For this review, take the finished solid that the model builds, in its own axes (mm). Face numbers are marked on the shaded views. A direction names the side the tool comes from. Give positions to 0.01 mm unless a question says otherwise; leave off trailing zeros. Order: outer loops, then holes, each group sorted by start corner. A loop starts at its lowest first (then second) coordinate and runs counter-clockwise, first axis right, second up. Notation, with made-up numbers: (-0.75, -1) - (14.25, -1) arc R8 cw to (14.25, 11) - close; hole circle Ø7 at (-2, 9). An arc over 180 degrees is marked (long way). Use a Markdown table: item, result. Add a question column.
1) We need section D-D on y = 2.5. Write out the cut boundary in (x, z).
2) We need section A-A on y = -52. Write out the cut boundary in (x, z).
3) Mouldability with a two-part tool opening along Y and no side actions: class the marked faces 1, 2 and 3 as released by +Y, released by -Y, zero draft, split by the parting line, or undercut.
4) Machinability: for the marked faces 4, 5 and 6, which of the approach directions +Z, -Z, +X, -X, +Y, -Y give a long, thin tool a straight path to every point of the face, cutting with its end or side? Answer none if there is none.
5) We need section C-C on z = 10.5. Write out the cut boundary in (x, y).
6) Wall thickness on L1, parallel to Y at x = 96.5, z = 22.5; L2, parallel to Y at x = 90.5, z = 23.5; L3, parallel to X at y = 152.5, z = 9.5: over which ranges is each line inside the solid? List them lowest first.
7) Clearance check with flat-ended pins moving along their axes: P1, Ø10, axis at y = 51, z = 108.5, coming from the +X side; P2, Ø1, axis at y = 103.5, z = 56, coming from the -X side; P3, Ø3, axis at x = 101.5, z = 52.5, coming from the -Y side; P4, Ø1.5, axis at x = 154.5, y = 118.5, coming from the +Z side. State where each tip first meets the part, or that it passes through.
8) We need section B-B on x = 114. Write out the cut boundary in (y, z), then the cut area to 3 significant figures.
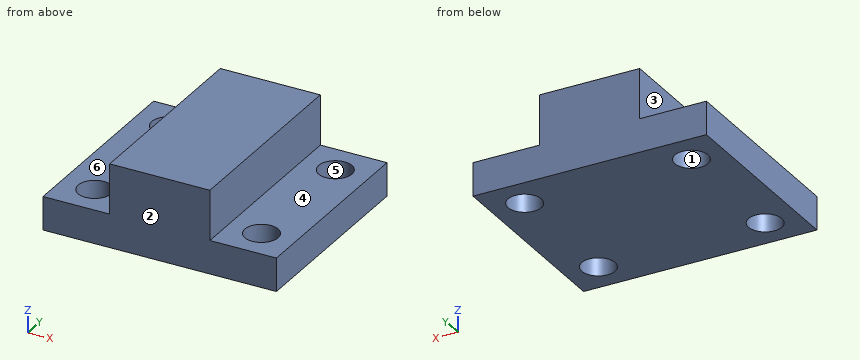
```python
from build123d import *

# Parameters (mm, degrees)
F1_DEPTH = 127
F0_W     = 101.6
F0_H     = 304.8
F0_R     = 25.4
F2_DEPTH = 50.8


with BuildPart() as f1:
    # F0 (on Top) → F1 (new body)
    with BuildSketch(Plane.XY):
        Polygon((308.34184, 208.50426), (155.882336, 208.50426), (155.882336, -96.29574), (308.49275, -96.29574), align=None)
    extrude(amount=F1_DEPTH)

    # F0 (on Top) → F2 (join)
    with BuildSketch(Plane.XY):
        with Locations((105.082336, 56.10426)):
            Rectangle(F0_W, F0_H)
        with Locations((105.082336, -45.49574)):
            Circle(F0_R, mode=Mode.SUBTRACT)
        with Locations((105.082336, 157.710619)):
            Circle(F0_R, mode=Mode.SUBTRACT)
        Polygon((308.34184, 208.50426), (155.882336, 208.50426), (155.882336, -96.29574), (308.49275, -96.29574), align=None)
        Polygon((409.882336, 208.50426), (308.34184, 208.50426), (308.49275, -96.29574), (409.882336, -96.29574), align=None)
        with Locations((359.175516, -45.538369)):
            Circle(F0_R, mode=Mode.SUBTRACT)
        with Locations((359.166974, 157.740726)):
            Circle(F0_R, mode=Mode.SUBTRACT)
    extrude(amount=F2_DEPTH)


solid = f1.part
```
Checked values:
| question | item | result |
|---|---|---|
| 1 | outline | (54.28, 0) - (409.88, 0) - (409.88, 50.8) - (308.44, 50.8) - (308.44, 127) - (155.88, 127) - (155.88, 50.8) - (54.28, 50.8) - close |
| 2 | outline | (54.28, 0) - (80.53, 0) - (80.53, 50.8) - (54.28, 50.8) - close; (129.64, 0) - (334.61, 0) - (334.61, 50.8) - (308.47, 50.8) - (308.47, 127) - (155.88, 127) - (155.88, 50.8) - (129.64, 50.8) - close; (383.74, 0) - (409.88, 0) - (409.88, 50.8) - (383.74, 50.8) - close |
| 3 | face 1 | undercut |
| 3 | face 2 | released by -Y |
| 3 | face 3 | zero draft |
| 4 | face 4 | +Z, +X, +Y, -Y |
| 4 | face 5 | +Z, -Z |
| 4 | face 6 | +Z, -X, +Y, -Y |
| 5 | outline | (54.28, -96.3) - (409.88, -96.3) - (409.88, 208.5) - (54.28, 208.5) - close; hole circle Ø50.8 at (105.08, -45.5); hole circle Ø50.8 at (105.08, 157.71); hole circle Ø50.8 at (359.17, 157.74); hole circle Ø50.8 at (359.18, -45.54) |
| 6 | L1 | -96.3 to -69.4, -21.59 to 133.8, 181.62 to 208.5 |
| 6 | L2 | -96.3 to -66.29, -24.7 to 136.91, 178.51 to 208.5 |
| 6 | L3 | 54.28 to 80.22, 129.94 to 334.31, 384.02 to 409.88 |
| 7 | P1 | x = 308.42 |
| 7 | P2 | x = 155.88 |
| 7 | P3 | through |
| 7 | P4 | z = 50.8 |
| 8 | outline | (-96.3, 0) - (-69.28, 0) - (-69.28, 50.8) - (-96.3, 50.8) - close; (-21.71, 0) - (133.93, 0) - (133.93, 50.8) - (-21.71, 50.8) - close; (181.49, 0) - (208.5, 0) - (208.5, 50.8) - (181.49, 50.8) - close |
| 8 | area | 10,700 mm² |
